Source: CAD feature listing. Evaluate the final solid. Frame: model axes, mm. A direction names the side the tool comes from. Give positions to 0.01 mm unless a question says otherwise; leave off trailing zeros. Order: outer loops, then holes, each group sorted by start corner. A loop starts at its lowest first (then second) coordinate and runs counter-clockwise, first axis right, second up. Notation, with made-up numbers: M 79,-6 L 127,-6 A7 cw 127,2 Z; hole C 14.25,62 d7. An arc over 180 degrees is marked long. Answer as a JSON object with one key per item and string values. Group by question number.
1. Material intervals for L1, parallel to Z at x = 19.5, y = -7; L2, parallel to X at y = -13, z = 18; L3, parallel to Y at x = -23, z = -31.5, sorted ascending. Write a range as [from, to].
2. Section query C-C (x = -25). Output: boundary loops of the cut face in (y, z), plus the area to 3 significant figures.
3. Section query B-B (z = 32). Output: boundary loops of the cut face in (x, y).
4. Set-up query: faces 1 (the flat face through (0, -13, -39.645)), 2 (the flat face through (0, -12, -41.645)). Return all of +Z, -Z, +X, -X, +Y, -Y with unobstructed straight access to the full face (end or side cutting, diameter ignored); none if empty.
5. Section query A-A (y = -7.5). Output: boundary loops of the cut face in (x, z).
from build123d import *

# Parameters (mm, degrees)
F0_W     = 62.305648
F0_H     = 83.289184
F0_W_2   = 58.305648
F0_H_2   = 79.289184
F1_DEPTH = 25
F2_DEPTH = 2
F3_W     = 58.305648
F3_H     = 1
F4_DEPTH = 23


with BuildPart() as f1:
    # F0 (on Front) → F1 (new body)
    with BuildSketch(Plane.XZ):
        Rectangle(F0_W, F0_H)
        Rectangle(F0_W_2, F0_H_2, mode=Mode.SUBTRACT)
    extrude(amount=F1_DEPTH)

    # F0 (on Front) → F2 (join)
    with BuildSketch(Plane.XZ):
        Rectangle(F0_W_2, F0_H_2)
    extrude(amount=F2_DEPTH)

    # F3 (on face) → F4 (join)
    with BuildSketch(Plane.XZ.offset(2)):
        with Locations((0, 24.144592)):
            Rectangle(F3_W, F3_H)
        with Locations((0, 9.144592)):
            Rectangle(F3_W, F3_H)
        with Locations((0, -6.855408)):
            Rectangle(F3_W, F3_H)
        with Locations((0, -22.855408)):
            Rectangle(F3_W, F3_H)
    extrude(amount=F4_DEPTH)


solid = f1.part
Answer sheet:
{
 "1": {"L1": "[-41.64, -39.64], [-23.36, -22.36], [-7.36, -6.36], [8.64, 9.64], [23.64, 24.64], [39.64, 41.64]", "L2": "[-31.15, -29.15], [29.15, 31.15]", "L3": "[-2, 0]"},
 "2": {"outline": "M -25,-41.64 L 0,-41.64 L 0,41.64 L -25,41.64 L -25,39.64 L -2,39.64 L -2,24.64 L -25,24.64 L -25,23.64 L -2,23.64 L -2,9.64 L -25,9.64 L -25,8.64 L -2,8.64 L -2,-6.36 L -25,-6.36 L -25,-7.36 L -2,-7.36 L -2,-22.36 L -25,-22.36 L -25,-23.36 L -2,-23.36 L -2,-39.64 L -25,-39.64 Z", "area": "351 mm^2"},
 "3": {"outline": "M -31.15,-25 L -29.15,-25 L -29.15,-2 L 29.15,-2 L 29.15,-25 L 31.15,-25 L 31.15,0 L -31.15,0 Z"},
 "4": {"face 1": "-Y", "face 2": "-Z, +X, -X, +Y, -Y"},
 "5": {"outline": "M -31.15,-41.64 L 31.15,-41.64 L 31.15,41.64 L -31.15,41.64 Z; hole M -29.15,-39.64 L 29.15,-39.64 L 29.15,-23.36 L -29.15,-23.36 Z; hole M -29.15,-22.36 L 29.15,-22.36 L 29.15,-7.36 L -29.15,-7.36 Z; hole M -29.15,-6.36 L 29.15,-6.36 L 29.15,8.64 L -29.15,8.64 Z; hole M -29.15,9.64 L 29.15,9.64 L 29.15,23.64 L -29.15,23.64 Z; hole M -29.15,24.64 L 29.15,24.64 L 29.15,39.64 L -29.15,39.64 Z"}
}
